The model under review builds one solid part; all positions refer to its coordinate system, in mm. A direction names the side the tool comes from. Coordinates: 2 decimals unless noted, no trailing zeros. Write each loop counter-clockwise with the first axis right and the second up, starting at its lowest first coordinate (ties: lowest second). Pieces come first, ordered by that corner, then holes. Notation, with made-up numbers: (-19, 69.5) - (1, 69.5) arc R26 cw to (1, 92.5) - close; hole circle Ø10 at (11.25, -29.5). An arc over 180 degrees is marked (long way). Return JSON: item names as keys, results as strings. Group by question number.
(1) We need section A-A on z = 19.5. State the section outline as (x, y) points, then the cut area to 3 significant figures.
(2) We need section C-C on y = 57. State the section outline as (x, z) points.
(3) We need section D-D on x = 0. State the section outline as (y, z) points.
(4) Tool access review of faces 1 (the face through (-20, 7, 31)), 2 (the face through (20, 7, 31)), 3 (the face through (27.436, 3.451, 39.976)): name each direction out of +Z, -Z, +X, -X, +Y, -Y from which nothing blocks a thin tool from reaching the whole face with its end or side.
(5) Draft analysis for pull direction X (two halves, no side actions). For faces 4 (the face through (27.17, 34.51, 3.45)), 5 (the face through (1, 30, 0)), 6 (the face through (-1.5, 78, 19)), state which applies: released by +X, released by -X, zero draft, split by the parting line, or undercut.
(6) To check wall thickness, follow L1, parallel to X at y = 1.75, z = 39; L2, parallel to Y at x = -7, z = 19; L3, parallel to Z at x = -5, y = 89. State the ranges of each line that lie inside material, in increasing order. Write a range as from..to.
(7) We need section B-B on x = 25.5. State the section outline as (y, z) points.
(8) For pin 1 Ø8 at (x, z) = (-3.5, 22) entering from -Y; pin 2 Ø7.5 at (x, y) = (-4.5, 83.5) entering from -Z; pin 3 Ø12 at (x, y) = (13, 20.5) entering from +Z; pin 4 Ø19 at (y, z) = (94, 14) entering from -X, all flat-tipped, find the tip position at first contact; note any pin that passes through.
```python
from build123d import *

# Parameters (mm, degrees)
SKETCH1_W                  = 72
SKETCH1_H                  = 7
BOSS_EXTRUDE1_DEPTH        = 55
BOSS_EXTRUDE2_DEPTH        = 7
BOSS_EXTRUDE3_DEPTH        = 39
BOSS_EXTRUDE4_START        = 7.5
BOSS_EXTRUDE4_DEPTH        = 24
BOSS_EXTRUDE5_DEPTH        = 55
FILLET3_RADIUS             = 12
FILLET3_LENGTH             = 7
FILLET4_RADIUS             = 12
FILLET4_LENGTH             = 7
CUT_EXTRUDE1_DEPTH         = 55
F_12_0MM_DOWEL_HOLE1_D     = 15
F_12_0MM_DOWEL_HOLE1_DEPTH = 30
F_12_0MM_DOWEL_HOLE1_TIP   = 4.506454643
FILLET5_R                  = 16
F_12_0MM_DOWEL_HOLE2_D     = 15
F_12_0MM_DOWEL_HOLE2_DEPTH = 30
F_12_0MM_DOWEL_HOLE2_TIP   = 4.506454643


with BuildPart() as part:
    # Sketch1 → Boss-Extrude1 (new body)
    with BuildSketch(Plane.XY):
        with Locations((0, 3.5)):
            Rectangle(SKETCH1_W, SKETCH1_H)
    extrude(amount=BOSS_EXTRUDE1_DEPTH)

    # Sketch1<3> → Boss-Extrude2 (add)
    with BuildSketch(Plane.XY):
        with BuildLine():
            Line((36, 7), (18.091261695, 62.805708421))
            ThreePointArc((18.091261695, 62.805708421), (16.449943687, 47.492142581), (4, 38.425824379))
            Line((4, 38.425824379), (4, 7))
            Line((4, 7), (36, 7))
        make_face()
        with BuildLine():
            ThreePointArc((-4, 38.425824379), (-16.449943687, 47.492142581), (-18.091261695, 62.805708421))
            Line((-18.091261695, 62.805708421), (-36, 7))
            Line((-36, 7), (-4, 7))
            Line((-4, 7), (-4, 38.425824379))
        make_face()
    extrude(amount=BOSS_EXTRUDE2_DEPTH)

    # Sketch1<4> → Boss-Extrude3 (add)
    with BuildSketch(Plane.XY):
        with BuildLine():
            ThreePointArc((-1.5, 68.9058809), (0, 45), (1.5, 68.9058809))
            Line((1.5, 68.9058809), (1.5, 75.940696925))
            ThreePointArc((1.5, 75.940696925), (0, 38), (-1.5, 75.940696925))
            Line((-1.5, 75.940696925), (-1.5, 68.9058809))
        make_face()
    extrude(amount=BOSS_EXTRUDE3_DEPTH)

    # Sketch1<5> → Boss-Extrude4 (add)
    with BuildSketch(Plane.XY.offset(BOSS_EXTRUDE4_START)):
        with BuildLine():
            Line((1.5, 101), (1.5, 75.940696925))
            ThreePointArc((1.5, 75.940696925), (5.093989215, 75.30440586), (8.5, 73.992645468))
            Line((8.5, 73.992645468), (8.5, 101))
            Line((8.5, 101), (1.5, 101))
        make_face()
        with BuildLine():
            ThreePointArc((-8.5, 73.992645468), (-5.093989215, 75.30440586), (-1.5, 75.940696925))
            Line((-1.5, 75.940696925), (-1.5, 101))
            Line((-1.5, 101), (-8.5, 101))
            Line((-8.5, 101), (-8.5, 73.992645468))
        make_face()
    extrude(amount=BOSS_EXTRUDE4_DEPTH)

    # Sketch1<6> → Boss-Extrude5 (add)
    with BuildSketch(Plane.XY):
        with BuildLine():
            ThreePointArc((4, 38.425824379), (0, 38), (-4, 38.425824379))
            Line((-4, 38.425824379), (-4, 7))
            Line((-4, 7), (4, 7))
            Line((4, 7), (4, 38.425824379))
        make_face()
    extrude(amount=BOSS_EXTRUDE5_DEPTH)

    # Fillet3: full round fillet: the end face becomes a half cylinder, R = half its width
    fillet3_face = Plane((5, 101, 19.5), x_dir=(1, 0, 0), z_dir=(0, 1, 0))  # on the end face: x along it, z out of the body
    fillet3_slab = fillet3_face.offset(-FILLET3_RADIUS / 2) * Box(FILLET3_LENGTH, 2 * FILLET3_RADIUS, FILLET3_RADIUS, mode=Mode.PRIVATE)  # the body's end, R deep
    fillet3_round = Plane((5, 89, 19.5), x_dir=(0, 1, 0), z_dir=(1, 0, 0)) * Cylinder(FILLET3_RADIUS, FILLET3_LENGTH, mode=Mode.PRIVATE)  # its axis R under the face
    add(fillet3_slab - fillet3_round, mode=Mode.SUBTRACT)

    # Fillet4: full round fillet: the end face becomes a half cylinder, R = half its width
    fillet4_face = Plane((-5, 101, 19.5), x_dir=(-1, 0, 0), z_dir=(0, 1, 0))  # on the end face: x along it, z out of the body
    fillet4_slab = fillet4_face.offset(-FILLET4_RADIUS / 2) * Box(FILLET4_LENGTH, 2 * FILLET4_RADIUS, FILLET4_RADIUS, mode=Mode.PRIVATE)  # the body's end, R deep
    fillet4_round = Plane((-5, 89, 19.5), x_dir=(0, 1, 0), z_dir=(-1, 0, 0)) * Cylinder(FILLET4_RADIUS, FILLET4_LENGTH, mode=Mode.PRIVATE)  # its axis R under the face
    add(fillet4_slab - fillet4_round, mode=Mode.SUBTRACT)

    # Sketch2 → Cut-Extrude1 (cut)
    with BuildSketch(Plane(origin=(4, 0, 0), x_dir=(0, 0, -1), z_dir=(1, 0, 0))):
        Polygon((-39, 38.425824379), (-55, 7), (-55, 38.425824379), align=None)
    extrude(amount=-CUT_EXTRUDE1_DEPTH, mode=Mode.SUBTRACT)

    # Ø12.0mm Dowel Hole1
    with Locations(Plane(origin=(8.5, 89, 19.5), x_dir=(0, 1, 0), z_dir=(1, 0, 0))):
        with Locations((0, 0)):
            Hole(F_12_0MM_DOWEL_HOLE1_D / 2, depth=F_12_0MM_DOWEL_HOLE1_DEPTH)
            with Locations((0, 0, -(F_12_0MM_DOWEL_HOLE1_DEPTH + F_12_0MM_DOWEL_HOLE1_TIP / 2))):  # 118° drill point
                Cone(0, F_12_0MM_DOWEL_HOLE1_D / 2, F_12_0MM_DOWEL_HOLE1_TIP, mode=Mode.SUBTRACT)

    # Fillet5
    fillet5_edges = [part.edges().sort_by_distance(p)[0] for p in [
        (-36, 3.5, 55),
        (36, 3.5, 55),
    ]]
    fillet(fillet5_edges, radius=FILLET5_R)

    # Ø12.0mm Dowel Hole2
    with Locations(Plane(origin=(20, 7, 39), x_dir=(0, 0, 1), z_dir=(0, 1, 0))):
        with Locations((0, 0), (0, -40)):
            Hole(F_12_0MM_DOWEL_HOLE2_D / 2, depth=F_12_0MM_DOWEL_HOLE2_DEPTH)
            with Locations((0, 0, -(F_12_0MM_DOWEL_HOLE2_DEPTH + F_12_0MM_DOWEL_HOLE2_TIP / 2))):  # 118° drill point
                Cone(0, F_12_0MM_DOWEL_HOLE2_D / 2, F_12_0MM_DOWEL_HOLE2_TIP, mode=Mode.SUBTRACT)


solid = part.part
```
Ans:
{
 "1": {"outline": "(-36, 0) - (36, 0) - (36, 7) - (4, 7) - (4, 38.43) arc R19 ccw to (8.5, 73.99) - (8.5, 81.5) - (1.5, 81.5) - (1.5, 68.91) arc R12 cw (long way) to (-1.5, 68.91) - (-1.5, 81.5) - (-8.5, 81.5) - (-8.5, 73.99) arc R19 ccw to (-4, 38.43) - (-4, 7) - (-36, 7) - close; (-8.5, 96.5) - (-1.5, 96.5) - (-1.5, 101) - (-8.5, 101) - close; (1.5, 96.5) - (8.5, 96.5) - (8.5, 101) - (1.5, 101) - close", "area": "1,560 mm²"},
 "2": {"outline": "(-19.95, 0) - (-12, 0) - (-12, 39) - (-19, 39) - (-19, 7) - (-19.95, 7) - close; (12, 0) - (19.95, 0) - (19.95, 7) - (19, 7) - (19, 39) - (12, 39) - close"},
 "3": {"outline": "(0, 0) - (45, 0) - (45, 39) - (38, 39) - (38, 39.22) - (7, 55) - (0, 55) - close"},
 "4": {"face 1": "+Z, -X", "face 2": "+Z, +X", "face 3": "-Y"},
 "5": {"face 4": "released by +X", "face 5": "zero draft", "face 6": "undercut"},
 "6": {"L1": "-36..-27.5, -12.5..12.5, 27.5..36", "L2": "0..7, 39.34..47.25, 66.75..81.52, 96.48..100.99", "L3": "7.5..12, 27..31.5"},
 "7": {"outline": "(0, 0) - (39.72, 0) - (39.72, 7) - (7, 7) - (7, 33.9) - (0, 33.9) - close; (0, 44.1) - (7, 44.1) - (7, 54.02) - (0, 54.02) - close"},
 "8": {"pin 1": "y = 0", "pin 2": "z = 7.5", "pin 3": "z = 7", "pin 4": "x = -8.5"}
}
